from build123d import *

# Parameters (mm, degrees)
F0_W     = 95.5
F0_H     = 64
F1_DEPTH = 2.5
F2_W     = 2.5
F2_H     = 64
F3_DEPTH = 20
F4_DEPTH = 70.5
F5_W     = 36
F5_H     = 2
F5_W_2   = 2
F5_H_2   = 21
F6_DEPTH = 5
F5_R     = 1.5
F7_DEPTH = 25


with BuildPart() as f1:
    # F0 (on Top) → F1 (new body)
    with BuildSketch(Plane.XY):
        with Locations((47.75, 32)):
            Rectangle(F0_W, F0_H)
    extrude(amount=F1_DEPTH)

    # F2 (on face) → F3 (join)
    with BuildSketch(Plane.XY.offset(2.5)):
        with Locations((1.25, 32)):
            Rectangle(F2_W, F2_H)
    extrude(amount=F3_DEPTH)

    # F2 (on face) → F4 (join)
    with BuildSketch(Plane.XY.offset(2.5)):
        with Locations((94.25, 32)):
            Rectangle(F2_W, F2_H)
    extrude(amount=F4_DEPTH)

    # F5 (on face) → F6 (join)
    with BuildSketch(Plane(origin=(93, 0, 0), x_dir=(0, -1, 0), z_dir=(-1, 0, 0))):
        with Locations((-32, 69.5)):
            Rectangle(F5_W, F5_H)
        with Locations((-8, 53)):
            Rectangle(F5_W_2, F5_H_2)
        with Locations((-32, 36.5)):
            Rectangle(F5_W, F5_H)
        with Locations((-56, 53)):
            Rectangle(F5_W_2, F5_H_2)
    extrude(amount=F6_DEPTH)

    # F5 (on face) → F7 (cut)
    with BuildSketch(Plane(origin=(93, 0, 0), x_dir=(0, -1, 0), z_dir=(-1, 0, 0))):
        with Locations((-35.5, 32.5)):
            Circle(F5_R)
        with Locations((-28.5, 32.5)):
            Circle(F5_R)
    extrude(amount=-F7_DEPTH, mode=Mode.SUBTRACT)


solid = f1.part
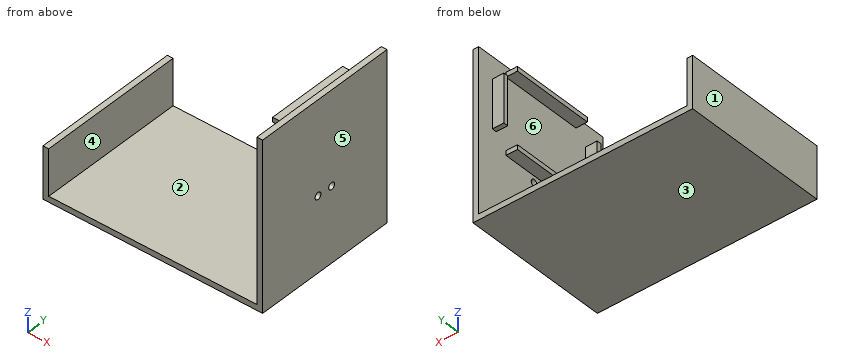
Could you check a few things on this model? Use its own coordinates, in mm. Face numbers are marked on the shaded views. A direction names the side the tool comes from. Give positions to 0.01 mm unless a question says otherwise; leave off trailing zeros. Order: outer loops, then holes, each group sorted by start corner. A loop starts at its lowest first (then second) coordinate and runs counter-clockwise, first axis right, second up. Notation, with made-up numbers: (0.25, 49) -> (5.25, 49) arc R12 ccw to (5.25, 59) -> close; hole circle Ø6 at (57, 55). An arc over 180 degrees is marked (long way). Return JSON: item names as keys, results as strings.
1. Thinking about a two-plate mould opening in X: for the marked faces 1, 2, 3 and 4, which applies, pulls with the +X half, pulls with the -X half, needs draft (parallel to the pull), parting line crosses it, or undercut?
Answer list:
{"face 1": "pulls with the -X half", "face 2": "undercut", "face 3": "needs draft", "face 4": "undercut"}
2. I need wall thicknesses on line 1 (Z direction, x = 89, y = 43.5); line 2 (X direction, y = 55, z = 11.5); line 3 (Z direction, x = 93.65, y = 35.5). Which ranges of each line are inside material? Lowest first, please. Write a range as from..to.
Answer list:
{"line 1": "z = 0..2.5, 35.5..37.5, 68.5..70.5", "line 2": "x = 0..2.5, 93..95.5", "line 3": "z = 0..31, 34..73"}
3. Imagine slicing it at C-C on y = 28.5. List the corners of the cut face in (x, z) for me.
Answer list:
{"outline": "(0, 0) -> (95.5, 0) -> (95.5, 31) -> (93, 31) -> (93, 2.5) -> (2.5, 2.5) -> (2.5, 22.5) -> (0, 22.5) -> close; (88, 35.5) -> (93, 35.5) -> (93, 34) -> (95.5, 34) -> (95.5, 73) -> (93, 73) -> (93, 70.5) -> (88, 70.5) -> (88, 68.5) -> (93, 68.5) -> (93, 37.5) -> (88, 37.5) -> close"}
4. Imagine slicing it at B-B on z = 32.5. List the corners of the cut face in (x, y) for me, then the cut area to 3 significant figures.
Answer list:
{"outline": "(93, 0) -> (95.5, 0) -> (95.5, 27) -> (93, 27) -> close; (93, 30) -> (95.5, 30) -> (95.5, 34) -> (93, 34) -> close; (93, 37) -> (95.5, 37) -> (95.5, 64) -> (93, 64) -> close", "area": "145 mm2"}
5. For pin 1 Ø2 at (y, z) = (39.5, 27.5) entering from -X; pin 2 Ø1.2 at (x, y) = (1.5, 47.5) entering from +Z; pin 3 Ø1.5 at (x, y) = (91, 25) entering from +Z; pin 4 Ø2 at (y, z) = (19, 18.5) entering from -X, each with a flat end and sliding along its axis, tell me the tip position at first contact or that it passes through.
Answer list:
{"pin 1": "stops at x = 93", "pin 2": "stops at z = 22.5", "pin 3": "stops at z = 70.5", "pin 4": "stops at x = 0"}
6. On a 3-axis mill with a long thin cutter (end or side, diameter ignored), from which of +Z, -Z, +X, -X, +Y, -Y can I reach the whole of each face in a straight line? I mean the marked faces 5 and 6. Say none if no direction works.
Answer list:
{"face 5": "+Z, -Z, +X, +Y, -Y", "face 6": "none"}
7. Imagine slicing it at A-A on z = 17.5. List the corners of the cut face in (x, y) for me.
Answer list:
{"outline": "(0, 0) -> (2.5, 0) -> (2.5, 64) -> (0, 64) -> close; (93, 0) -> (95.5, 0) -> (95.5, 64) -> (93, 64) -> close"}
8. Imagine slicing it at D-D on z = 49. List the corners of the cut face in (x, y) for me, then the cut area to 3 significant figures.
Answer list:
{"outline": "(88, 7) -> (93, 7) -> (93, 0) -> (95.5, 0) -> (95.5, 64) -> (93, 64) -> (93, 57) -> (88, 57) -> (88, 55) -> (93, 55) -> (93, 9) -> (88, 9) -> close", "area": "180 mm2"}
